Input: dimensioned drawing with shaded views. Units: mm. Origin: part minimum x, y, z. Round coordinates to 2 decimals unless told otherwise and drop trailing zeros. Order: outer loops, then holes, each group sorted by start corner. A loop starts at its lowest first (then second) coordinate and runs counter-clockwise, first axis right, second up. Notation, with made-up numbers: M -5,30 L 12,30 A13 cw 12,41 Z; hole C 16.25,-22 d7. An arc over 180 degrees is marked long. One line per question, with ' | ' between items.
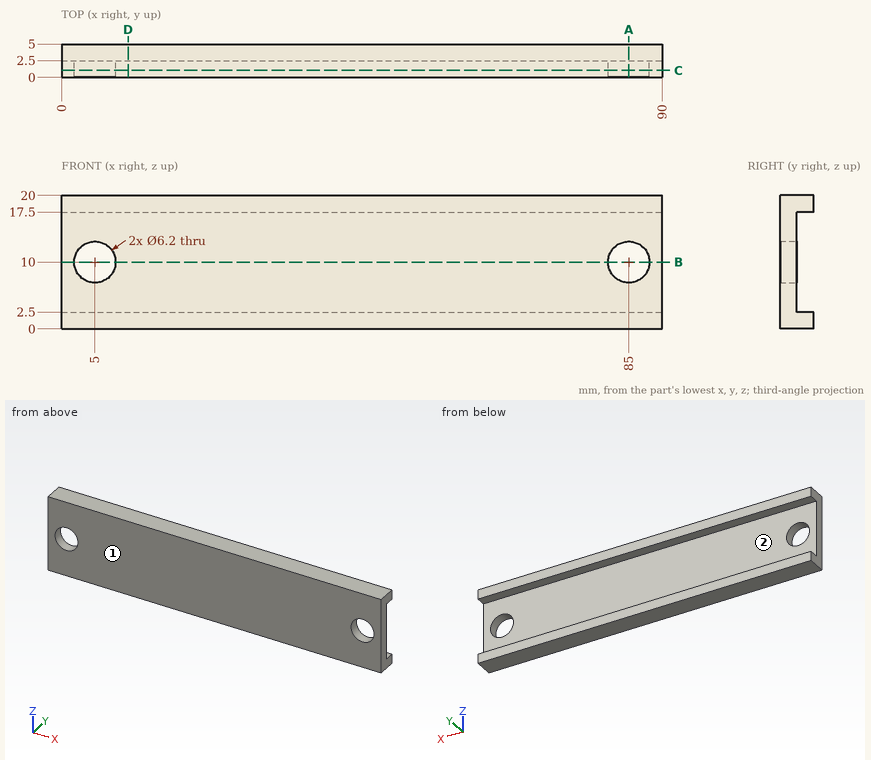
Item 1: Section query A-A, the plane x = 85. Return loops of the section in (y, z), plus the area to 3 significant figures.
Report:
outline: M 0,0 L 5,0 L 5,2.5 L 2.5,2.5 L 2.5,6.9 L 0,6.9 Z; M 0,13.1 L 2.5,13.1 L 2.5,17.5 L 5,17.5 L 5,20 L 0,20 Z | area: 47.0 mm²
Item 2: Mould query, pull axis Z, two halves, no side actions, for the marked faces 1 and 2. Classes: +Z half, -Z half, draft (parallel to the pull), parting line (faces both ways), or undercut.
Report:
face 1: draft | face 2: undercut
Item 3: Section query B-B, the plane z = 10. Return loops of the section in (x, y), plus the area to 3 significant figures.
Report:
outline: M 0,0 L 1.9,0 L 1.9,2.5 L 0,2.5 Z; M 8.1,0 L 81.9,0 L 81.9,2.5 L 8.1,2.5 Z; M 88.1,0 L 90,0 L 90,2.5 L 88.1,2.5 Z | area: 194 mm²
Item 4: Section query C-C, the plane y = 1.05. Return loops of the section in (x, z).
Report:
outline: M 0,0 L 90,0 L 90,20 L 0,20 Z; hole C 5,10 d6.2; hole C 85,10 d6.2
Item 5: First-contact query: pin 1 (10 mm diameter, centred on x = 23, z = 9.5, fed in from +Y). Flat tip, straight axial feed; report the tip coordinate or a pass-through.
Report:
pin 1: y = 2.5
Item 6: Line query: line 1 along Z through (x, y) = (5, 0.6); line 2 along Z through (x, y) = (13.5, 3); line 3 along Y through (x, z) = (85, 3). Output: solid intervals per line, ascending. Write a range as from..to.
Report:
line 1: 0..6.9, 13.1..20 | line 2: 0..2.5, 17.5..20 | line 3: 0..2.5
Item 7: Section query D-D, the plane x = 10. Return loops of the section in (y, z).
Report:
outline: M 0,0 L 5,0 L 5,2.5 L 2.5,2.5 L 2.5,17.5 L 5,17.5 L 5,20 L 0,20 Z
